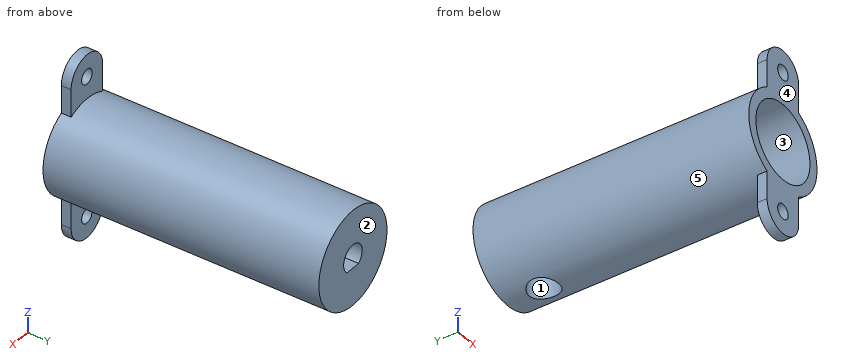
Autodesk Inventor part; units mm, degrees
ref_plane "Work Plane1" through (0, 0, -9.7) normal (0, 0, 1) x (1, 0, 0)
ref_plane "YZ Plane" through (0, 0, 0) normal (1, 0, 0) x (0, 1, 0)
ref_plane "XZ Plane" through (0, 0, 0) normal (0, 1, 0) x (-1, 0, 0)
sketch "Sketch1" plane through (0, 0, 0) normal (0, 1, 0) x (-1, 0, 0)
  line L0 (0, 0) -> (4.8, 0) construction
  circle A0 centre (0, 0) radius 2.5 construction
  circle A1 centre (0, 0) radius 2.65
  line L1 (0.0078, 2.5) -> (0.0078, -2.1) construction
  line L2 (0.0078, 2.5) -> (4.6078, 2.5) construction
  line L3 (0.0078, -2.1) -> (1.6163, -2.1)
  line L4 (0.0078, -2.1) -> (-1.6163, -2.1)
  line L5 (0.0078, -2.1) -> (1.6319, -2.1) construction
  circle A2 centre (0, 0) radius 7.5 construction
  circle A3 centre (0, 0) radius 7.7
  circle A4 centre (0, 0) radius 9.7
  dimension "d5" = 5
  dimension "d6" = 0.15
  dimension "d7" = 4.6
  dimension "d8" = 90
  dimension "d9" = 90
  dimension "d10" = 180
  dimension "d26" = 15
  dimension "d27" = 0.2
  dimension "d28" = 2
extrude "Extrusion5" add sketch "Sketch1" along normal blind 16 contours L4 L3 A1 | A3 | A4 picked at (-0.9103, -2.2002)
extrude "Extrusion6" add sketch "Sketch1" along normal blind 1 contours A1 L3 L4 picked at (0.0374, 1.0538)
extrude "Extrusion7" add sketch "Sketch1" against normal blind 40 contours A4
ref_plane "Work Plane1" through (0, 0, -9.7) normal (0, 0, 1) x (1, 0, 0)
sketch "Sketch3" plane through (0, 0, -9.7) normal (0, 0, 1) x (1, 0, 0)
  circle A0 centre (0, 8.5) radius 1.5
  circle A1 centre (0, 8.5) radius 3
  point P0 (0, 0)
  dimension "d35" = 3
  dimension "d36" = 6
extrude "Extrusion8" cut sketch "Sketch3" along normal blind 7.7 contours A0
extrude "Extrusion9" cut sketch "Sketch3" along normal blind 10
sketch "Sketch4" plane through (0, -40, 0) normal (0, -1, 0) x (1, 0, 0)
  circle A0 centre (0, 0) radius 9.7
  circle A1 centre (0, 14.2) radius 1.5
  line L0 (0, 12.7) -> (0, 9.7) construction
  circle A2 centre (0, 14.2) radius 4.5
  line L1 (4.5, 14.2) -> (4.5, 8.593)
  line L2 (-4.5, 14.2) -> (-4.5, 8.593)
  circle A3 centre (0, 0) radius 9.7
  dimension "d42" = 3
  dimension "d43" = 3
  dimension "d44" = 3
extrude "Extrusion10" add sketch "Sketch4" against normal blind 2 contours A0 A2 L1 | L2 A2 A0 | A2
pattern_circular "Circular Pattern1" count 2 over 360 about axis through (0, 0, 0) along (0, -1, 0) of "Extrusion10"
properties part number "Arm"
Part model, mm, in its own coordinate system. Face numbers are marked on the shaded views. A direction names the side the tool comes from. Coordinates: 2 decimals unless noted, no trailing zeros. Order: outer loops, then holes, each group sorted by start corner. A loop starts at its lowest first (then second) coordinate and runs counter-clockwise, first axis right, second up. Notation, with made-up numbers: (70.5, 84) -> (115.5, 84) arc R10 ccw to (115.5, 102) -> close; hole circle Ø5 at (39, 55). An arc over 180 degrees is marked (long way). Put each result on its own line as item: value. Start each with the question number.
(1) Band-saw the part on C-C (y = -31). Give the cut face in (x, z), then the cut area to 3 significant figures.
(2) Mould opens along Y. For the marked faces 1, 2 and 3 say: pulls with the +Y half, pulls with the -Y half, needs draft (parallel to the pull), parting line crosses it, or undercut.
(3) Band-saw the part on A-A (x = 0). Give the cut face in (y, z).
(4) Band-saw the part on B-B (z = -4). Give the cut face in (x, y), then the cut area to 3 significant figures.
(5) Which spindle directions (+Z, -Z, +X, -X, +Y, -Y) get a long thin tool onto all of the face, cutting with end or side? Do the marked faces 4 and 5. Say none if no direction does.
(6) Band-saw the part on D-D (x = 7). Give the cut face in (y, z).
(7) Probe line 1 along Z through (x, y) = (0, -39.4); line 2 along X through (y, z) = (10, 0); line 3 along Y through (x, z) = (0, -7). List the from-to ranges inside material, lowest first. Write a range as [from, to].
(8) Pin check, flat tips, straight feed: pin 1 Ø2 at (x, z) = (6.5, 13) entering from -Y; pin 2 Ø10 at (y, z) = (-4, -0.5) entering from -X; pin 3 Ø10 at (y, z) = (-12, -8) entering from +X; pin 4 Ø4.5 at (x, z) = (2, 1) entering from -Y. Stop position of each tip, or through.
Determined:
1. outline: circle Ø19.4 at (0, 0); hole circle Ø15.4 at (0, 0)
1. area: 109 mm²
2. face 1: undercut
2. face 2: pulls with the +Y half
2. face 3: needs draft
3. outline: (-40, -18.7) -> (-38, -18.7) -> (-38, -15.7) -> (-40, -15.7) -> close; (-40, -12.7) -> (-38, -12.7) -> (-38, -9.7) -> (5.5, -9.7) -> (5.5, -2.1) -> (1, -2.1) -> (1, 2.65) -> (16, 2.65) -> (16, 9.7) -> (-38, 9.7) -> (-38, 12.7) -> (-40, 12.7) -> (-40, 7.7) -> (0, 7.7) -> (0, -7.7) -> (-40, -7.7) -> close; (-40, 15.7) -> (-38, 15.7) -> (-38, 18.7) -> (-40, 18.7) -> close; (11.5, -9.7) -> (16, -9.7) -> (16, -2.1) -> (11.5, -2.1) -> close
4. outline: (-8.84, -40) -> (-6.58, -40) -> (-6.58, 0) -> (6.58, 0) -> (6.58, -40) -> (8.84, -40) -> (8.84, 16) -> (-8.84, 16) -> close; hole circle Ø6 at (0, 8.5)
4. area: 435 mm²
5. face 4: +Z, -Z, +X, -X, -Y
5. face 5: +Y
6. outline: (-40, -6.71) -> (16, -6.71) -> (16, 6.71) -> (-40, 6.71) -> (-40, 3.21) -> (0, 3.21) -> (0, -3.21) -> (-40, -3.21) -> close
7. line 1: z = [-18.7, -15.7], [-12.7, -7.7], [7.7, 12.7], [15.7, 18.7]
7. line 2: x = [-9.7, -2.65], [2.65, 9.7]
7. line 3: y = [0, 5.5], [11.5, 16]
8. pin 1: passes through
8. pin 2: stops at x = -9.7
8. pin 3: stops at x = 9.22
8. pin 4: stops at y = 0
